For this review, use the dimensioned drawing (mm, ordinates from the lowest corner) and the shaded views. Give positions to 0.01 mm unless a question says otherwise; leave off trailing zeros. Order: outer loops, then holes, each group sorted by start corner. A loop starts at its lowest first (then second) coordinate and runs counter-clockwise, first axis right, second up. Notation, with made-up numbers: (55.5, -31.5) -> (83.5, -31.5) arc R23 cw to (83.5, -22.5) -> close; hole circle Ø4 at (34.5, 46.5). An arc over 180 degrees is marked (long way). Return JSON: item names as keys, results as strings.
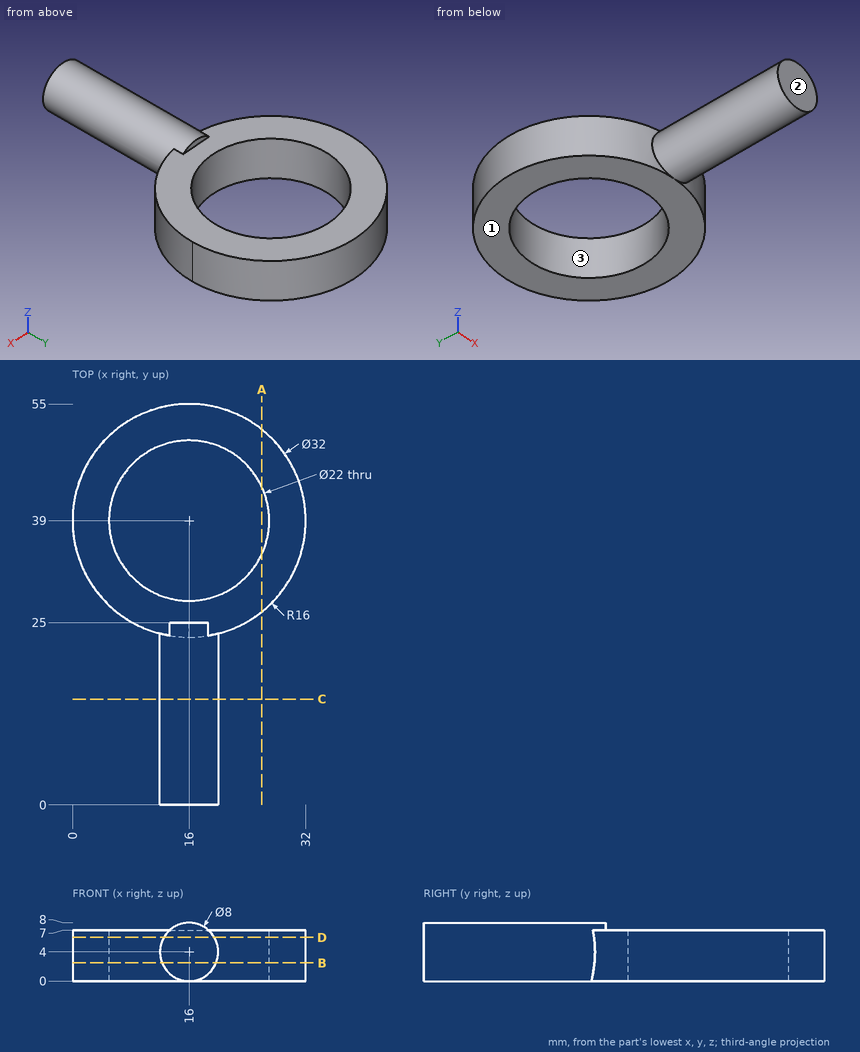
Item 1: Add section A-A (x = 26). Give the boundary of the cut face in (y, z).
Result set:
{"outline": "(26.51, 0) -> (34.42, 0) -> (34.42, 7) -> (26.51, 7) -> close; (43.58, 0) -> (51.49, 0) -> (51.49, 7) -> (43.58, 7) -> close"}
Item 2: Add section D-D (z = 6). Give the boundary of the cut face in (x, y).
Result set:
{"outline": "(12.54, 0) -> (19.46, 0) -> (19.46, 23.38) arc R16 ccw (long way) to (12.54, 23.38) -> close; hole circle Ø22 at (16, 39)"}
Item 3: Wall thickness on L1, parallel to Y at x = 16, z = 2.5; L2, parallel to Y at x = 19.5, z = 3; L3, parallel to X at y = 33, z = 3.75: over which ranges is each line inside the solid? List them lowest first. Write a range as [from, to].
Result set:
{"L1": "y = [0, 28], [50, 55]", "L2": "y = [0, 28.57], [49.43, 54.61]", "L3": "x = [1.17, 6.78], [25.22, 30.83]"}
Item 4: Add section B-B (z = 2.5). Give the boundary of the cut face in (x, y), plus the area to 3 significant figures.
Result set:
{"outline": "(12.29, 0) -> (19.71, 0) -> (19.71, 23.44) arc R16 ccw (long way) to (12.29, 23.44) -> close; hole circle Ø22 at (16, 39)", "area": "596 mm^2"}
Item 5: Mouldability with a two-part tool opening along Y and no side actions: class the marked faces 1, 2 and 3 as released by +Y, released by -Y, zero draft, split by the parting line, or undercut.
Result set:
{"face 1": "zero draft", "face 2": "released by -Y", "face 3": "undercut"}
Item 6: For pin 1 (1.1 mm diameter, centred on x = 16, z = 7.5, fed in from +Y); pin 2 (12 mm diameter, centred on x = 17, y = 44, fed in from +Z); pin 3 (3 mm diameter, centred on y = 21.5, z = 3.5, fed in from +X); pin 4 (4 mm diameter, centred on y = 15.5, z = 5, fed in from -X), all flat-tipped, find the tip position at first contact; note any pin that passes through.
Result set:
{"pin 1": "stops at y = 55", "pin 2": "stops at z = 7", "pin 3": "stops at x = 20", "pin 4": "stops at x = 12"}
Item 7: Add section C-C (y = 14.5). Give the boundary of the cut face in (x, z), plus the area to 3 significant figures.
Result set:
{"outline": "circle Ø8 at (16, 4)", "area": "50.3 mm^2"}
